Input: part model. Units: mm. Frame: model coordinates. Coordinates: 2 decimals unless noted, no trailing zeros. Loops run counter-clockwise (first coordinate to the right, second up) from the corner with the lowest first, then second, coordinate; pieces in that order, holes last.
```python
from build123d import *

# Parameters (mm, degrees)
SKETCH1_W                    = 57.15
SKETCH1_H                    = 15.875
BOSS_EXTRUDE1_DEPTH          = 3.175
F_0_257_DIAMETER_HOLE1_D     = 6.5278
FILLET1_R                    = 6.35
F_18_0_1695_DIAMETER_HOLE1_D = 4.3053


with BuildPart() as part:
    # Sketch1 → Boss-Extrude1 (new body)
    with BuildSketch(Plane(origin=(0, 0, 0), x_dir=(1, 0, 0), z_dir=(0, 1, 0))):
        Rectangle(SKETCH1_W, SKETCH1_H)
    extrude(amount=BOSS_EXTRUDE1_DEPTH)

    # F (0.257) Diameter Hole1 (through all)
    with Locations(Plane(origin=(0, 3.175, 0), x_dir=(1, 0, 0), z_dir=(0, 1, 0))):
        with Locations((-19.05, 0)):
            Hole(F_0_257_DIAMETER_HOLE1_D / 2)

    # Fillet1
    fillet1_edges = [part.edges().sort_by_distance(p)[0] for p in [
        (-28.575, 1.5875, 7.9375),
        (-28.575, 1.5875, -7.9375),
    ]]
    fillet(fillet1_edges, radius=FILLET1_R)

    # #18 (0.1695) Diameter Hole1 (through all)
    with Locations(Plane(origin=(0, 3.175, 0), x_dir=(1, 0, 0), z_dir=(0, 1, 0))):
        with Locations((-6.35, 0), (6.35, 0)):
            Hole(F_18_0_1695_DIAMETER_HOLE1_D / 2)


solid = part.part
```
Item 1: Line query: L1, parallel to Z at x = 6.35, y = 2; L2, parallel to X at y = 2.5, z = 1.25 (3 decimals); L3, parallel to X at y = 0.85, z = 0.5 (3 decimals). Output: solid intervals per line, ascending.
Result:
L1: z = -7.94 to -2.15, 2.15 to 7.94
L2: x = -28.575 to -22.065, -16.035 to -8.103, -4.597 to 4.597, 8.103 to 28.575
L3: x = -28.575 to -22.275, -15.825 to -8.444, -4.256 to 4.256, 8.444 to 28.575
Item 2: Section query C-C (z = -0.75). Output: boundary loops of the cut face in (x, y) (3 decimals).
Result:
outline: (-28.575, 0) - (-22.227, 0) - (-22.227, 3.175) - (-28.575, 3.175) - close; (-15.873, 0) - (-8.368, 0) - (-8.368, 3.175) - (-15.873, 3.175) - close; (-4.332, 0) - (4.332, 0) - (4.332, 3.175) - (-4.332, 3.175) - close; (8.368, 0) - (28.575, 0) - (28.575, 3.175) - (8.368, 3.175) - close
Item 3: Section query D-D (x = 6.35). Output: boundary loops of the cut face in (y, z) (1 decimal), then the cut area to 3 significant figures.
Result:
outline: (0, -7.9) - (3.2, -7.9) - (3.2, -2.2) - (0, -2.2) - close; (0, 2.2) - (3.2, 2.2) - (3.2, 7.9) - (0, 7.9) - close
area: 36.7 mm2
Item 4: Section query A-A (y = 1.35). Count the separate pieces of the cut face and the enclosed holes in it, then the cut area to 3 significant figures.
Result:
separate pieces: 1
enclosed holes: 3
area: 827 mm2
Item 5: Section query B-B (x = -19.05). Output: boundary loops of the cut face in (y, z) (1 decimal), then the cut area to 3 significant figures.
Result:
outline: (0, -7.9) - (3.2, -7.9) - (3.2, -3.3) - (0, -3.3) - close; (0, 3.3) - (3.2, 3.3) - (3.2, 7.9) - (0, 7.9) - close
area: 29.7 mm2
Item 6: Mould query, pull axis Z, two halves, no side actions, for faces 1 (the face through (3, 2, -7.938)), 2 (the face through (-4.2, 1.6, -0.1)), 3 (the face through (3, 2, 7.938)), 4 (the face through (0, 3.175, 0)). Classes: +Z half, -Z half, draft (parallel to the pull), parting line (faces both ways), or undercut.
Result:
face 1: -Z half
face 2: undercut
face 3: +Z half
face 4: draft
